Design review of the part built by this model. Coordinates are the model's own, in mm. A direction names the side the tool comes from. Give positions to 0.01 mm unless a question says otherwise; leave off trailing zeros. Loops run counter-clockwise (first coordinate to the right, second up) from the corner with the lowest first, then second, coordinate; pieces in that order, holes last. Notation, with made-up numbers: (65, 73) - (111, 73) arc R27 ccw to (111, 109) - close; hole circle Ø9 at (11, 89.5). An arc over 180 degrees is marked (long way). Write each question's results on one line, items separated by ' | '.
```python
from build123d import *

# Parameters (mm, degrees)
F0_W     = 6.35
F0_H     = 6.35
F1_DEPTH = 6.35
F2_W     = 3.589511
F2_H     = 3.439947
F3_DEPTH = 2.54
F4_W     = 3.589511
F4_H     = 3.439947
F5_DEPTH = 2.54
F7_D     = 3.81


with BuildPart() as f1:
    # F0 (on Right) → F1 (new body)
    with BuildSketch(Plane.YZ):
        with Locations((-38.814982, 3.175)):
            Rectangle(F0_W, F0_H)
    extrude(amount=F1_DEPTH)



with BuildPart() as f3:
    # F2 (on face) → F3 (new body)
    with BuildSketch(Plane.YZ.offset(8.89)):
        with Locations((-38.873002, 3.177181)):
            Rectangle(F2_W, F2_H)
    extrude(amount=F3_DEPTH)


with BuildPart() as f1_1:
    add(f1.part)

    add(f3.part)  # F5 merges F3
    # F4 (on face) → F5 (join)
    with BuildSketch(Plane.YZ.offset(6.35)):
        with Locations((-38.873002, 3.177181)):
            Rectangle(F4_W, F4_H)
    extrude(amount=F5_DEPTH)

    # F7 (through all)
    with Locations(Plane.XZ.offset(40.667757)):
        with Locations((8.89, 4.897155)):
            Hole(F7_D / 2)


solid = f1_1.part
```
Item 1: We need section A-A on z = 2. Give the boundary of the cut face in (x, y).
Output values:
outline: (0, -41.99) - (6.35, -41.99) - (6.35, -40.67) - (11.43, -40.67) - (11.43, -37.08) - (6.35, -37.08) - (6.35, -35.64) - (0, -35.64) - close
Item 2: We need section D-D on x = 8.89. Give the boundary of the cut face in (y, z).
Output values:
outline: (-40.67, 1.46) - (-37.08, 1.46) - (-37.08, 2.99) - (-40.67, 2.99) - close
Item 3: Draft analysis for pull direction X (two halves, no side actions). For faces 5 (the face through (3, -35.64, 3)), 6 (the face through (8.932, -38.848, 2.993)), 7 (the face through (0, -39, 3)), 8 (the face through (11.43, -39, 3)), state which applies: +X half, -X half, draft (parallel to the pull), parting line (faces both ways), or undercut.
Output values:
face 5: draft | face 6: undercut | face 7: -X half | face 8: +X half
Item 4: We need section B-B on y = -37.5. Give the boundary of the cut face in (x, z) (3 decimals), then the cut area to 3 significant figures.
Output values:
outline: (0, 0) - (6.35, 0) - (6.35, 1.457) - (11.43, 1.457) - (11.43, 4.897) - (10.795, 4.897) arc R1.905 cw to (6.985, 4.897) - (6.35, 4.897) - (6.35, 6.35) - (0, 6.35) - close | area: 52.1 mm²
Item 5: Clearance check with flat-ended pins moving along their axes: P1, Ø3, axis at x = 9.5, z = 3, coming from the +Y side; P2, Ø1.8, axis at x = 9, y = -39.5, coming from the -Z side; P3, Ø1.7, axis at x = 10, z = 2.5, coming from the -Y side. State where each tip first meets the part, or that it passes through.
Output values:
P1: stops at y = -37.08 | P2: stops at z = 1.46 | P3: stops at y = -40.67
Item 6: Tool access review of faces 1 (the face through (8.9, -40.668, 2.8)), 2 (the face through (8.9, -37.078, 2.8)), 3 (the face through (3, -39, 6.35)), 4 (the face through (9, -39, 1.457)): name each direction out of +Z, -Z, +X, -X, +Y, -Y from which nothing blocks a thin tool from reaching the whole face with its end or side.
Output values:
face 1: +Z, -Z, +X, -Y | face 2: +Z, -Z, +X, +Y | face 3: +Z, +X, -X, +Y, -Y | face 4: -Z, +X, +Y, -Y
Item 7: We need section C-C on z = 3.75. Give the boundary of the cut face in (x, y).
Output values:
outline: (0, -41.99) - (6.35, -41.99) - (6.35, -40.67) - (7.37, -40.67) - (7.37, -37.08) - (6.35, -37.08) - (6.35, -35.64) - (0, -35.64) - close; (10.41, -40.67) - (11.43, -40.67) - (11.43, -37.08) - (10.41, -37.08) - close
Item 8: Wall thickness on probe 1 along X at (y, z) = (-40.75, 1.5); probe 2 along X at (y, z) = (-38, 4.75); probe 3 along X at (y, z) = (-39.25, 4.25): over which ranges is each line inside the solid? List them lowest first.
Output values:
probe 1: x = 0 to 6.35 | probe 2: x = 0 to 6.99, 10.79 to 11.43 | probe 3: x = 0 to 7.1, 10.68 to 11.43
